Source: three-view drawing plus pictorial views. Frame: mm from the lowest corner of the part. A direction names the side the tool comes from. Round coordinates to 2 decimals unless told otherwise and drop trailing zeros. Write each loop counter-clockwise with the first axis right and the second up, starting at its lowest first coordinate (ties: lowest second). Pieces come first, ordered by that corner, then holes. Notation, with made-up numbers: (-7, -24) -> (27, -24) arc R17 ccw to (27, 0) -> close; hole circle Ø11 at (-25, -14). An arc over 180 degrees is marked (long way). Put each result on its own line as item: value.
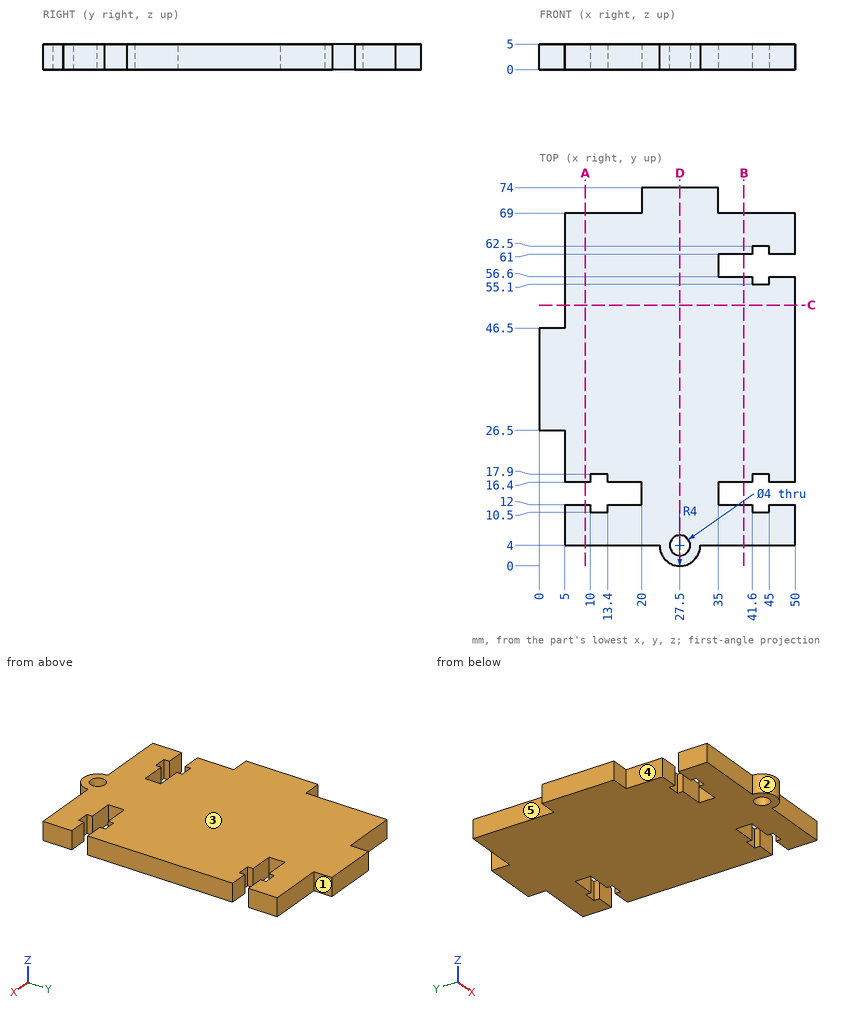
Q1. Cut plane A-A on x = 9. Output: boundary loops of the cut face in (y, z).
Ans:
outline: (4, 0) -> (12, 0) -> (12, 5) -> (4, 5) -> close; (16.4, 0) -> (69, 0) -> (69, 5) -> (16.4, 5) -> close
Q2. Reachability of the marked faces 1, 2, 3, 4 and 5 from +Z, -Z, +X, -X, +Y, -Y: full face, straight path, thin tool, end or side. Return the list, or none.
Ans:
face 1: +Z, -Z, +X, +Y
face 2: +Z, -Z, -Y
face 3: +Z, +X, -X, +Y, -Y
face 4: +Z, -Z, -X, -Y
face 5: +Z, -Z, -X, +Y
Q3. Material intervals for line 1 (Y direction, x = 37, z = 2.35); line 2 (Y direction, x = 43, z = 1.5); line 3 (Y direction, x = 27.5, z = 4.6), sorted ascending. Write a range as [from, to].
Ans:
line 1: y = [4, 12], [16.4, 56.6], [61, 69]
line 2: y = [4, 10.5], [17.9, 55.1], [62.5, 69]
line 3: y = [0, 2], [6, 74]
Q4. Cut plane C-C on y = 51. Output: boundary loops of the cut face in (x, z).
Ans:
outline: (5, 0) -> (50, 0) -> (50, 5) -> (5, 5) -> close
Q5. Pin query (flat end, axial travel): pin 1 (0.8 mm diameter, centred on y = 56, z = 3.5, fed in from -X); pin 2 (1.5 mm diameter, centred on x = 40, z = 2, fed in from +Y); pin 3 (1.7 mm diameter, centred on x = 11, z = 3.5, fed in from -Y). Return the tip coordinate at first contact, or that it passes through.
Ans:
pin 1: stops at x = 5
pin 2: stops at y = 69
pin 3: stops at y = 4
Q6. Cut plane D-D on x = 27.5. Output: boundary loops of the cut face in (y, z), and give its area (3 significant figures).
Ans:
outline: (0, 0) -> (2, 0) -> (2, 5) -> (0, 5) -> close; (6, 0) -> (74, 0) -> (74, 5) -> (6, 5) -> close
area: 350 mm^2
Q7. Cut plane B-B on x = 40. Output: boundary loops of the cut face in (y, z).
Ans:
outline: (4, 0) -> (12, 0) -> (12, 5) -> (4, 5) -> close; (16.4, 0) -> (56.6, 0) -> (56.6, 5) -> (16.4, 5) -> close; (61, 0) -> (69, 0) -> (69, 5) -> (61, 5) -> close
